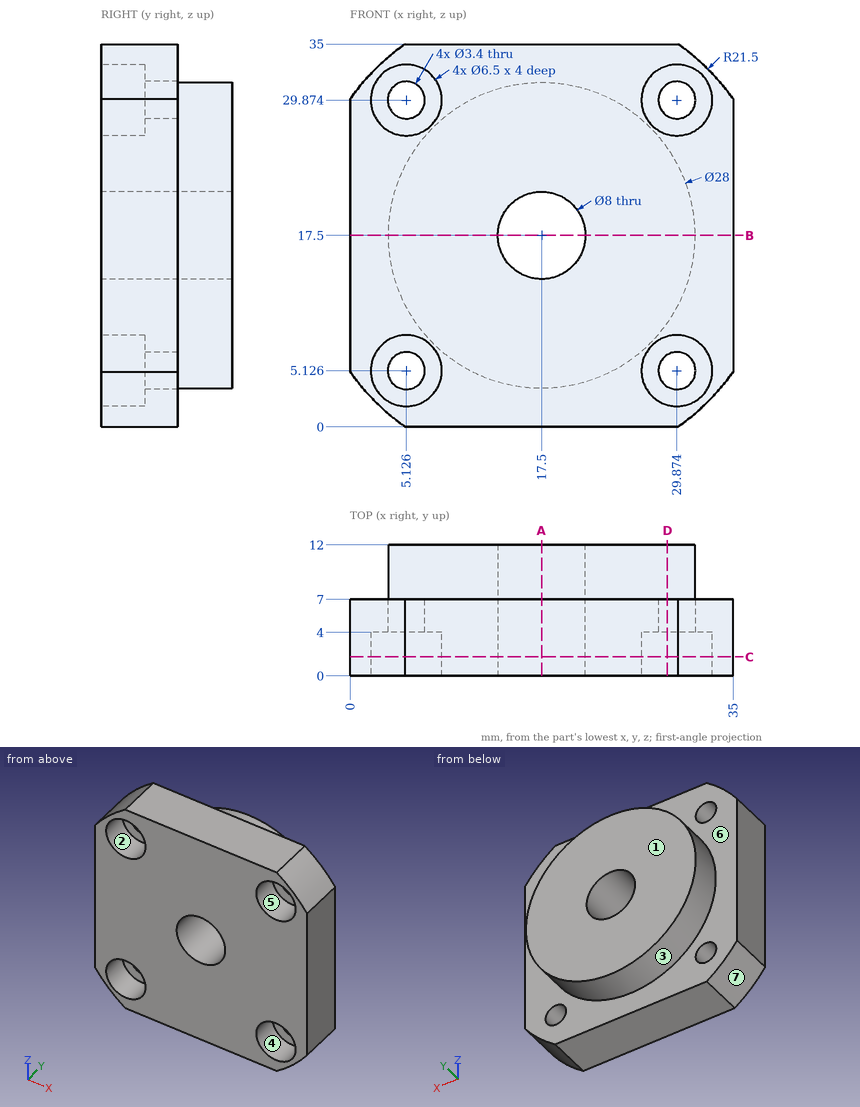
Geometry: see drawing. Coordinates: mm, zero at the bounding-box minimum. A direction names the side the tool comes from. Give positions to 0.01 mm unless a question says otherwise; leave off trailing zeros. Order: outer loops, then holes, each group sorted by start corner. A loop starts at its lowest first (then second) coordinate and runs counter-clockwise, first axis right, second up. Notation, with made-up numbers: M -26,83.5 L -4,83.5 A15 ccw -4,99.5 Z; hole C -37.75,55 d1. An arc over 180 degrees is marked long. Answer as CSV lines item,"result". Start each with the question number.
1) Line query: line 1 (X direction, y = 9, z = 17.5); line 2 (X direction, y = 2.25, z = 2.5) (1 decimal); line 3 (X direction, y = 5, z = 30). Output: solid intervals per line, ascending. Write a range as from..to.
2) First-contact query: P1, Ø4.5, axis at x = 5.13, z = 5.13, coming from the -Y side; P2, Ø5.5, axis at x = 29.87, z = 5.13, coming from the +Y side; P3, Ø7, axis at x = 6.5, z = 29, coming from the -Y side. Flat tips, straight axial feed; report the tip coordinate or a pass-through.
3) Cut plane B-B (z = 17.5). Output: boundary loops of the cut face in (x, y), then the cut area to 3 significant figures.
4) Cut plane C-C (y = 1.75). State how many separate pieces and enclosed holes the cut face has.
5) Cut plane D-D (x = 29). Output: boundary loops of the cut face in (y, z) (1 decimal).
6) Mould query, pull axis Z, two halves, no side actions, for the marked faces 1, 2, 3 and 4. Classes: +Z half, -Z half, draft (parallel to the pull), parting line (faces both ways), or undercut.
7) Set-up query: the marked faces 5, 6 and 7. Return all of +Z, -Z, +X, -X, +Y, -Y with unobstructed straight access to the full face (end or side cutting, diameter ignored); none if empty.
8) Cut plane A-A (x = 17.5). Output: boundary loops of the cut face in (y, z).
Findings below:
1,line 1,"x = 3.5..13.5, 21.5..31.5"
1,line 2,"x = 2.1..3.2, 7..28, 31.8..32.9"
1,line 3,"x = 0.01..3.43, 6.82..28.18, 31.57..34.99"
2,P1,"stops at y = 4"
2,P2,"stops at y = 7"
2,P3,"stops at y = 0"
3,outline,"M 0,0 L 13.5,0 L 13.5,12 L 3.5,12 L 3.5,7 L 0,7 Z; M 21.5,0 L 35,0 L 35,7 L 31.5,7 L 31.5,12 L 21.5,12 Z"
3,area,"289 mm²"
4,separate pieces,"1"
4,enclosed holes,"5"
5,outline,"M 0,0 L 7,0 L 7,3.7 L 4,3.7 L 4,2 L 0,2 Z; M 0,8.3 L 4,8.3 L 4,6.6 L 7,6.6 L 7,9.5 L 12,9.5 L 12,25.5 L 7,25.5 L 7,28.4 L 4,28.4 L 4,26.7 L 0,26.7 Z; M 0,33 L 4,33 L 4,31.3 L 7,31.3 L 7,35 L 0,35 Z"
6,face 1,"draft"
6,face 2,"undercut"
6,face 3,"parting line"
6,face 4,"undercut"
7,face 5,"-Y"
7,face 6,"+Y"
7,face 7,"-Z, -X, +Y, -Y"
8,outline,"M 0,0 L 7,0 L 7,3.5 L 12,3.5 L 12,13.5 L 0,13.5 Z; M 0,21.5 L 12,21.5 L 12,31.5 L 7,31.5 L 7,35 L 0,35 Z"
